Geometry: see drawing. Coordinates: mm, zero at the bounding-box minimum. A direction names the side the tool comes from. Coordinates: 2 decimals unless noted, no trailing zeros. Loops run counter-clockwise (first coordinate to the right, second up) from the corner with the lowest first, then second, coordinate; pieces in that order, holes last. Notation, with made-up numbers: (-3.75, 53.5) - (44.25, 53.5) arc R16 cw to (44.25, 83.5) - close; hole circle Ø4 at (9.25, -31.5). An arc over 180 degrees is marked (long way). Write item = value, one per line. Start each with the question number.
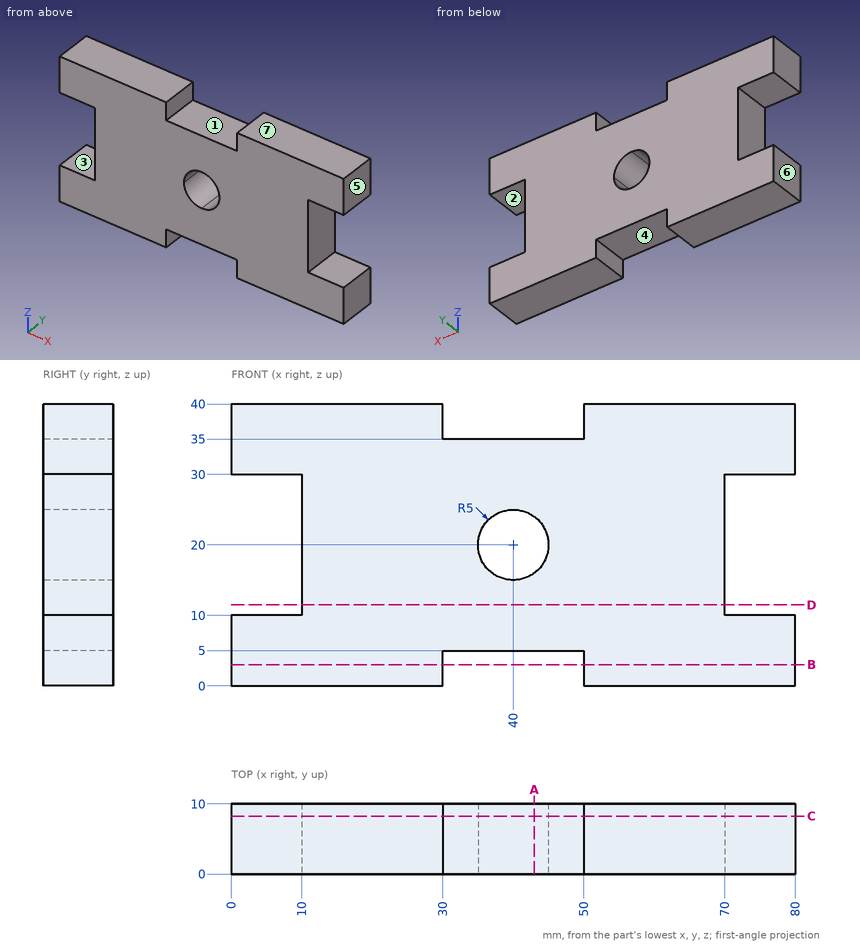
Item 1: First-contact query: pin 1 (6 mm diameter, centred on y = 6, z = 26.5, fed in from +X); pin 2 (2 mm diameter, centred on y = 4, z = 19.5, fed in from -X). Flat tips, straight axial feed; report the tip coordinate or a pass-through.
Item 2: Draft query along X for the marked faces 4, 5, 6 and 7. Return one class per face: released by +X, released by -X, zero draft, split by the parting line, or undercut.
Item 3: Cut plane D-D (z = 11.5). Return the cut outline in (x, y), then the cut area to 3 significant figures.
Item 4: Cut plane B-B (z = 3). Return the cut outline in (x, y), then the cut area to 3 significant figures.
Item 5: Cut plane A-A (x = 43). Return the cut outline in (y, z).
Item 6: Material intervals for L1, parallel to Z at x = 9.5, y = 9.5; L2, parallel to X at y = 5.5, z = 20; L3, parallel to X at y = 8.25, z = 37, sorted ascending. Write a range as [from, to].
Item 7: Reachability of the marked faces 1, 2 and 3 from +Z, -Z, +X, -X, +Y, -Y: full face, straight path, thin tool, end or side. Return the list, or none.
Item 8: Cut plane C-C (y = 8.25). Return the cut outline in (x, z), then the cut area to 3 significant figures.
Responses:
q1.pin_1 = 70
q1.pin_2 = 10
q2.face_4 = undercut
q2.face_5 = released by +X
q2.face_6 = released by -X
q2.face_7 = zero draft
q3.outline = (10, 0) - (70, 0) - (70, 10) - (10, 10) - close
q3.area = 600 mm2
q4.outline = (0, 0) - (30, 0) - (30, 10) - (0, 10) - close; (50, 0) - (80, 0) - (80, 10) - (50, 10) - close
q4.area = 600 mm2
q5.outline = (0, 5) - (10, 5) - (10, 16) - (0, 16) - close; (0, 24) - (10, 24) - (10, 35) - (0, 35) - close
q6.L1 = [0, 10], [30, 40]
q6.L2 = [10, 35], [45, 70]
q6.L3 = [0, 30], [50, 80]
q7.face_1 = +Z, +Y, -Y
q7.face_2 = +X, +Y, -Y
q7.face_3 = -X, +Y, -Y
q8.outline = (0, 0) - (30, 0) - (30, 5) - (50, 5) - (50, 0) - (80, 0) - (80, 10) - (70, 10) - (70, 30) - (80, 30) - (80, 40) - (50, 40) - (50, 35) - (30, 35) - (30, 40) - (0, 40) - (0, 30) - (10, 30) - (10, 10) - (0, 10) - close; hole circle Ø10 at (40, 20)
q8.area = 2,520 mm2
